from build123d import *

# Parameters (mm, degrees)
SKETCH_1_R          = 50
EXTRUDE_1_DEPTH     = 1150
CUT_EXTRUDE_1_DEPTH = 100
SKETCH_3_R          = 30
CUT_EXTRUDE_2_DEPTH = 100
SKETCH_4_R          = 50
CUT_EXTRUDE_3_DEPTH = 100
SKETCH_6_R          = 72.906400888
CUT_EXTRUDE_4_DEPTH = 50
SCALE_1_SCALE       = 0.345


with BuildPart() as part:
    # 草图1 → 凸台-拉伸1 (new body)
    with BuildSketch(Plane.XY):
        Circle(SKETCH_1_R)
    extrude(amount=EXTRUDE_1_DEPTH)

    # 草图2 → 切除-拉伸1 (cut)
    with BuildSketch(Plane.XY.offset(1150)):
        Polygon((-30, 50), (-30, -50), (-82.719574124, -32.427051987), (-69.504020862, 45.153140313), align=None)
        Polygon((30, 50), (30, -50), (70.972415669, -45.887337717), (95.445662451, 11.135327286), align=None)
    extrude(amount=-CUT_EXTRUDE_1_DEPTH, mode=Mode.SUBTRACT)

    # 草图3 → 切除-拉伸2 (cut)
    with BuildSketch(Plane(origin=(30, 0, 0), x_dir=(0, 0, -1), z_dir=(1, 0, 0))):
        with Locations((-1100, 0)):
            Circle(SKETCH_3_R)
    extrude(amount=-CUT_EXTRUDE_2_DEPTH, mode=Mode.SUBTRACT)

    # 圆角1: read off the stored shape, not the designer's step
    # 圆角1 outline → 圆角1 (revolve, cut)
    with BuildSketch(Plane.XZ):
        with BuildLine():
            ThreePointArc((0, 1150), (35.355339077, 1135.355339042), (50, 1099.99999995))
            Line((50, 1099.99999995), (50, 1150))
            Line((50, 1150), (0, 1150))
        make_face()
    revolve(axis=Axis((0, 0, 0), (0, 0, 1)), mode=Mode.SUBTRACT)

    # 草图4 → 切除-拉伸3 (cut)
    with BuildSketch(Plane(origin=(0, 0, 0), x_dir=(-1, 0, 0), z_dir=(0, 0, -1))):
        Circle(SKETCH_4_R)
    extrude(amount=-CUT_EXTRUDE_3_DEPTH, mode=Mode.SUBTRACT)

    # 草图6 → 切除-拉伸4 (cut)
    with BuildSketch(Plane(origin=(0, 0, 100), x_dir=(-1, 0, 0), z_dir=(0, 0, -1))):
        Circle(SKETCH_6_R)
    extrude(amount=-CUT_EXTRUDE_4_DEPTH, mode=Mode.SUBTRACT)


with BuildPart() as part_1:
    # 缩放比例1: scaled about (0, 0, 0)
    add(part.part.scale(SCALE_1_SCALE))


solid = part_1.part
Design review of the part built by this model. Coordinates are the model's own, in mm. A direction names the side the tool comes from. Round coordinates to 2 decimals unless told otherwise and drop trailing zeros. Write each loop counter-clockwise with the first axis right and the second up, starting at its lowest first coordinate (ties: lowest second). Pieces come first, ordered by that corner, then holes.
Item 1: Wall thickness on L1, parallel to X at y = 1, z = 86; L2, parallel to X at y = -11, z = 382: over which ranges is each line inside the solid? List them lowest first.
Item 2: Draft analysis for pull direction Y (two halves, no side actions). For faces 4 (the cylindrical face through (0.145, -3.964, 369.939)), 5 (the cylindrical face through (16.453, 5.181, 213.331)), 6 (the flat face through (-13, 0, 362.25)), state which applies: released by +Y, released by -Y, zero draft, split by the parting line, or undercut.
Item 3: Consider section B-B on y = 7.5. Give the boundary of the cut face in (x, z).
Item 4: For pin 1 Ø1.5 at (x, z) = (9, 100.5) entering from +Y; pin 2 Ø1.5 at (x, z) = (10, 323) entering from +Y; pin 3 Ø3 at (x, y) = (6, 2.5) entering from +Z; pin 4 Ø12.5 at (y, z) = (0, 379.5) entering from -X, all flat-tipped, find the tip position at first contact; note any pin that passes through.
Item 5: For faces 1 (the flat face through (0, 0, 51.75)), 2 (the flat face through (-10.35, 6.33, 371.09)), 3 (the flat face through (10.35, 6.33, 371.09)), list the 3-axis set-ups (+Z, -Z, +X, -X, +Y, -Y) from which the entire face can be reached by the end or side of a thin tool; tool diameter is ignored.
Item 6: Consider section C-C on z = 341.5. Give the boundary of the cut face in (x, y), and give its area (3 significant figures).
Item 7: Consider section A-A on x = 0. Give the boundary of the cut face in (y, z), and give its area (3 significant figures).
Check values:
1. L1: x = -17.22 to 17.22
1. L2: x = -10.35 to 10.35
2. face 4: undercut
2. face 5: split by the parting line
2. face 6: zero draft
3. outline: (-15.53, 51.75) - (15.53, 51.75) - (15.53, 362.25) - (10.35, 362.25) - (10.35, 372.37) - (-10.35, 372.37) - (-10.35, 362.25) - (-15.53, 362.25) - close; (-10.35, 386.63) - (10.35, 386.63) - (10.35, 391.08) arc R15.53 ccw to (-10.35, 391.08) - close
4. pin 1: stops at y = 15.15
4. pin 2: stops at y = 14.56
4. pin 3: stops at z = 396.01
4. pin 4: passes through
5. face 1: -Z, +X, -X, +Y, -Y
5. face 2: +Z, -X, +Y, -Y
5. face 3: +Z, +X, +Y, -Y
6. outline: circle Ø34.5 at (0, 0)
6. area: 935 mm2
7. outline: (-17.25, 51.75) - (17.25, 51.75) - (17.25, 379.5) arc R17.25 ccw to (-17.25, 379.5) - close; hole circle Ø20.7 at (0, 379.5)
7. area: 11,400 mm2
